For this review, take the finished solid that the model builds, in its own axes (mm). A direction names the side the tool comes from. Round coordinates to 2 decimals unless told otherwise and drop trailing zeros. Order: outer loops, then holes, each group sorted by start corner. A loop starts at its lowest first (then second) coordinate and runs counter-clockwise, first axis right, second up.
Autodesk Inventor part; units mm, degrees
ref_plane "YZ Plane" through (0, 0, 0) normal (1, 0, 0) x (0, 1, 0)
ref_plane "XZ Plane" through (0, 0, 0) normal (0, 1, 0) x (-1, 0, 0)
ref_plane "XY Plane" through (0, 0, 0) normal (0, 0, 1) x (1, 0, 0)
sketch "Sketch2" plane through (0, 0, 0) normal (1, 0, 0) x (0, 1, 0)
  line L0 (-7.5, 4.3301) -> (0, 8.6603)
  line L1 (0, 8.6603) -> (7.5, 4.3301)
  line L2 (7.5, 4.3301) -> (7.5, -4.3301)
  line L3 (7.5, -4.3301) -> (0, -8.6603)
  line L4 (0, -8.6603) -> (-7.5, -4.3301)
  line L5 (-7.5, -4.3301) -> (-7.5, 4.3301)
  line L6 (0, 12.1244) -> (0, -12.1244)
  circle A0 centre (0, 0) radius 5
  dimension "d1" = 10
extrude "Extrusion1" add sketch "Sketch2" along normal blind 11.4 contours L0 L6 A0 L4 L5 | L1 L2 L3 L6 A0
sketch "Sketch3" plane through (0, 0, 0) normal (0, 0, 1) x (1, 0, 0)
  line L0 (0, 10.9) -> (0, -10.9)
  line L1 (0, -10.9) -> (0, -5)
  line L2 (0, -10.9) -> (1.5, -10.9)
  line L3 (1.5, -10.9) -> (3.9439, -5)
  line L4 (3.9439, -5) -> (0, -5)
  line L5 (-0.7888, 0) -> (4.7326, 0)
  point P0 (0, 0)
  dimension "d4" = 1.5
  dimension "d5" = 22.5
  dimension "d6" = 5
revolve "Revolution1" add sketch "Sketch3" angle 360 about axis through (0, 0, 0) along (1, 0, 0)
sketch "Sketch4" plane through (0, 0, 0) normal (0, 1, 0) x (-1, 0, 0)
  line L0 (-11.4, 4.3301) -> (-11.4, 8.6603)
  line L1 (-11.4, 6.36) -> (-10.26, 6.36)
  line L2 (-10.26, 6.36) -> (-9.12, 7.5)
  line L3 (-9.12, 7.5) -> (-8.0461, 9.36)
  line L4 (-8.0461, 9.36) -> (-11.4, 9.36)
  line L5 (-11.4, 9.36) -> (-11.4, 6.36)
  line L6 (-9.12, 7.5) -> (-10.26, 6.36)
  line L7 (-8.4501, 8.6603) -> (-9.12, 7.5)
  line L8 (2.28, 0) -> (-13.68, 0)
  point P0 (0, 0)
  dimension "d8" = 135
  dimension "d9" = 1.14
  dimension "d10" = 6.36
  dimension "d11" = 120
  dimension "d12" = 2.28
  dimension "d13" = 3
revolve "Revolution2" cut sketch "Sketch4" angle 360 about axis through (-10, 0, 0) along (1, 0, 0)
thread "Thread1"
properties part number "314-11" material "Steel, Mild"
(1) Add section B-B on x = 8.75. Give the boundary of the cut face in (y, z), plus the area to 3 significant figures.
(2) Draft analysis for pull direction Z (two halves, no side actions). For faces 1 (the face through (0, 2, -5)), 2 (the face through (5.727, -3.802, 6.465)), 3 (the face through (8.96, 0.02, -7.78)), 4 (the face through (5.62, -1.08, 4.88)), state which applies: pulls with the +Z half, pulls with the -Z half, needs draft (parallel to the pull), parting line crosses it, or undercut.
(3) Tool access review of faces 5 (the face through (5.727, 3.802, -6.465)), 6 (the face through (5.727, 3.697, 6.526)), 7 (the face through (5.727, -3.697, -6.526)): name each direction out of +Z, -Z, +X, -X, +Y, -Y from which nothing blocks a thin tool from reaching the whole face with its end or side.
(4) Clearance check with flat-ended pins moving along their axes: P1, Ø1, axis at x = 8.5, z = -8, coming from the -Y side; P2, Ø3.5, axis at x = 6.5, z = 0, coming from the -Y side; P3, Ø5.5, axis at x = 6, z = 1, coming from the +Y side. State where each tip first meets the part, or that it passes through.
(5) Add section C-C on x = 1. Give the boundary of the cut face in (y, z).
(6) Wall thickness on L1, parallel to Y at x = 5, z = 0; L2, parallel to Z at x = 9, y = -2; L3, parallel to Z at x = 0.5, y = 1.25: over which ranges is each line inside the solid? List them lowest first.
(7) Add section A-A on x = 3.5. Give the boundary of the cut face in (y, z).
Here are the results:
1. outline: (-7.5, -3.17) arc R8.14 ccw to (-6.49, -4.91) - (-1.01, -8.08) arc R8.14 ccw to (1.01, -8.08) - (6.49, -4.91) arc R8.14 ccw to (7.5, -3.17) - (7.5, 3.17) arc R8.14 ccw to (6.49, 4.91) - (1.01, 8.08) arc R8.14 ccw to (-1.01, 8.08) - (-6.49, 4.91) arc R8.14 ccw to (-7.5, 3.17) - close; hole circle Ø10 at (0, 0)
1. area: 113 mm2
2. face 1: needs draft
2. face 2: pulls with the +Z half
2. face 3: pulls with the -Z half
2. face 4: undercut
3. face 5: -Z, +X, +Y
3. face 6: +Z, +X, +Y
3. face 7: -Z, +X, -Y
4. P1: stops at y = -2.01
4. P2: stops at y = -7.5
4. P3: stops at y = 7.5
5. outline: circle Ø21.8 at (0, 0); hole circle Ø10 at (0, 0)
6. L1: y = -7.5 to -5, 5 to 7.5
6. L2: z = -7.44 to -4.58, 4.58 to 7.44
6. L3: z = -10.83 to -4.84, 4.84 to 10.83
7. outline: (-7.5, -4.33) - (0, -8.66) - (7.5, -4.33) - (7.5, 4.33) - (0, 8.66) - (-7.5, 4.33) - close; hole circle Ø10 at (0, 0)
